from build123d import *

# Parameters (mm, degrees)
CUT_EXTRUDE_START           = 11
CUT_EXTRUDE_1_OUTLINE_R     = 2.9
CUT_EXTRUDE_1_DEPTH         = 5
CUT_EXTRUDE_1_2_OUTLINE_R   = 2.9
CUT_EXTRUDE_1_2_DEPTH       = 4.9999999
CUT_EXTRUDE_START_2         = 2
CUT_EXTRUDE_1_3_OUTLINE_R   = 2.9
CUT_EXTRUDE_1_3_OUTLINE_R_2 = 1.6
CUT_EXTRUDE_1_3_DEPTH       = 12
CUT_EXTRUDE_START_3         = 4.9999999
CUT_EXTRUDE_1_4_OUTLINE_R   = 2.9
CUT_EXTRUDE_1_4_DEPTH       = 6.0000001
CUT_EXTRUDE_START_4         = 15.5
CUT_EXTRUDE_1_5_OUTLINE_R   = 5.75
CUT_EXTRUDE_1_5_OUTLINE_R_2 = 3
CUT_EXTRUDE_1_5_DEPTH       = 1.5
CUT_EXTRUDE_START_5         = 14
CUT_EXTRUDE_1_6_OUTLINE_R   = 4
CUT_EXTRUDE_1_6_OUTLINE_R_2 = 3
CUT_EXTRUDE_1_6_DEPTH       = 1.5
CUT_EXTRUDE_1_7_OUTLINE_R   = 3
CUT_EXTRUDE_1_7_DEPTH       = 14
CUT_EXTRUDE_START_6         = 14.5
CUT_EXTRUDE_1_8_OUTLINE_R   = 3
CUT_EXTRUDE_1_8_DEPTH       = 14
SKETCH_2_R                  = 6.172348418
CUT_EXTRUDE_2_DEPTH         = 3
SKETCH_3_R                  = 1.803021439
CUT_EXTRUDE_3_DEPTH         = 10
SM_BASE_FLANGE_1_DEPTH      = 16
SKETCH_7_R                  = 1.782386215
EXTRUDE_1_DEPTH             = 25
SKETCH_8_R                  = 3.028561668
EXTRUDE_2_DEPTH             = 5
CUT_EXTRUDE_4_DEPTH         = 4
EXTRUDE_3_DEPTH             = 3
SKETCH_11_R                 = 2.38049646
EXTRUDE_4_DEPTH             = 10


with BuildPart() as part:
    # Cut-Extrude 1: read off the stored shape, not the designer's step
    # Cut-Extrude 1 outline → Cut-Extrude 1 (new body)
    with BuildSketch(Plane(origin=(0, 0, 0), x_dir=(1, 0, 0), z_dir=(0, 1, 0)).offset(CUT_EXTRUDE_START)):
        with BuildLine():
            ThreePointArc((-12, 28.5), (-13.414213562, 27.914213562), (-14, 26.5))
            Line((-14, 26.5), (-14, -26.5))
            ThreePointArc((-14, -26.5), (-13.414213562, -27.914213562), (-12, -28.5))
            Line((-12, -28.5), (12, -28.5))
            ThreePointArc((12, -28.5), (13.414213562, -27.914213562), (14, -26.5))
            Line((14, -26.5), (14, 26.5))
            ThreePointArc((14, 26.5), (13.414213562, 27.914213562), (12, 28.5))
            Line((12, 28.5), (-12, 28.5))
        make_face()
        with Locations((9, -23.5)):
            Circle(CUT_EXTRUDE_1_OUTLINE_R, mode=Mode.SUBTRACT)
        with Locations((9, 23.5)):
            Circle(CUT_EXTRUDE_1_OUTLINE_R, mode=Mode.SUBTRACT)
    extrude(amount=CUT_EXTRUDE_1_DEPTH)



with BuildPart() as body_2:
    # Cut-Extrude 1 2 outline → Cut-Extrude 1 2 (new body)
    with BuildSketch(Plane(origin=(0, 0, 0), x_dir=(1, 0, 0), z_dir=(0, 1, 0))):
        with BuildLine():
            ThreePointArc((-12, 28.5), (-13.414213562, 27.914213562), (-14, 26.5))
            Line((-14, 26.5), (-14, -26.5))
            ThreePointArc((-14, -26.5), (-13.414213562, -27.914213562), (-12, -28.5))
            Line((-12, -28.5), (12, -28.5))
            ThreePointArc((12, -28.5), (13.414213562, -27.914213562), (14, -26.5))
            Line((14, -26.5), (14, 26.5))
            ThreePointArc((14, 26.5), (13.414213562, 27.914213562), (12, 28.5))
            Line((12, 28.5), (-12, 28.5))
        make_face()
        with Locations((9, -23.5)):
            Circle(CUT_EXTRUDE_1_2_OUTLINE_R, mode=Mode.SUBTRACT)
        with Locations((9, 23.5)):
            Circle(CUT_EXTRUDE_1_2_OUTLINE_R, mode=Mode.SUBTRACT)
    extrude(amount=CUT_EXTRUDE_1_2_DEPTH)


with BuildPart() as part_1:
    add(part.part)

    add(body_2.part)  # Cut-Extrude 1 3 merges body 2
    # Cut-Extrude 1 3 outline → Cut-Extrude 1 3 (add)
    # profile 1 of 2: a face of its own
    with BuildSketch(Plane(origin=(0, 0, 0), x_dir=(1, 0, 0), z_dir=(0, 1, 0)).offset(CUT_EXTRUDE_START_2)):
        with Locations((9, 23.5)):
            Circle(CUT_EXTRUDE_1_3_OUTLINE_R)
        with Locations((9, 23.5)):
            Circle(CUT_EXTRUDE_1_3_OUTLINE_R_2, mode=Mode.SUBTRACT)
    # profile 2 of 2: a face of its own
    with BuildSketch(Plane(origin=(0, 0, 0), x_dir=(1, 0, 0), z_dir=(0, 1, 0)).offset(CUT_EXTRUDE_START_2)):
        with Locations((9, -23.5)):
            Circle(CUT_EXTRUDE_1_3_OUTLINE_R)
        with Locations((9, -23.5)):
            Circle(CUT_EXTRUDE_1_3_OUTLINE_R_2, mode=Mode.SUBTRACT)
    extrude(amount=CUT_EXTRUDE_1_3_DEPTH)

    # Cut-Extrude 1 4 outline → Cut-Extrude 1 4 (add)
    with BuildSketch(Plane(origin=(0, 0, 0), x_dir=(1, 0, 0), z_dir=(0, 1, 0)).offset(CUT_EXTRUDE_START_3)):
        with BuildLine():
            ThreePointArc((-12, 28.5), (-13.414213562, 27.914213562), (-14, 26.5))
            Line((-14, 26.5), (-14, -26.5))
            ThreePointArc((-14, -26.5), (-13.414213562, -27.914213562), (-12, -28.5))
            Line((-12, -28.5), (12, -28.5))
            ThreePointArc((12, -28.5), (13.414213562, -27.914213562), (14, -26.5))
            Line((14, -26.5), (14, 26.5))
            ThreePointArc((14, 26.5), (13.414213562, 27.914213562), (12, 28.5))
            Line((12, 28.5), (-12, 28.5))
        make_face()
        with Locations((9, -23.5)):
            Circle(CUT_EXTRUDE_1_4_OUTLINE_R, mode=Mode.SUBTRACT)
        with Locations((9, 23.5)):
            Circle(CUT_EXTRUDE_1_4_OUTLINE_R, mode=Mode.SUBTRACT)
    extrude(amount=CUT_EXTRUDE_1_4_DEPTH)



with BuildPart() as body_2_2:
    # Cut-Extrude 1 5 outline → Cut-Extrude 1 5 (new body)
    with BuildSketch(Plane.YZ.offset(CUT_EXTRUDE_START_4)):
        with Locations((8, 7.5)):
            Circle(CUT_EXTRUDE_1_5_OUTLINE_R)
        with Locations((8, 7.5)):
            Circle(CUT_EXTRUDE_1_5_OUTLINE_R_2, mode=Mode.SUBTRACT)
    extrude(amount=CUT_EXTRUDE_1_5_DEPTH)


with BuildPart() as part_2:
    add(part_1.part)

    add(body_2_2.part)  # Cut-Extrude 1 6 merges body 2 2
    # Cut-Extrude 1 6 outline → Cut-Extrude 1 6 (add)
    with BuildSketch(Plane.YZ.offset(CUT_EXTRUDE_START_5)):
        with Locations((8, 7.5)):
            Circle(CUT_EXTRUDE_1_6_OUTLINE_R)
        with Locations((8, 7.5)):
            Circle(CUT_EXTRUDE_1_6_OUTLINE_R_2, mode=Mode.SUBTRACT)
    extrude(amount=CUT_EXTRUDE_1_6_DEPTH)

    # Cut-Extrude 1 7 outline → Cut-Extrude 1 7 (cut)
    with BuildSketch(Plane.YZ):
        with Locations((8, 7.5)):
            Circle(CUT_EXTRUDE_1_7_OUTLINE_R)
    extrude(amount=CUT_EXTRUDE_1_7_DEPTH, mode=Mode.SUBTRACT)

    # Cut-Extrude 1 8 outline → Cut-Extrude 1 8 (cut)
    with BuildSketch(Plane.XY.offset(CUT_EXTRUDE_START_6)):
        with Locations((-5, 8)):
            Circle(CUT_EXTRUDE_1_8_OUTLINE_R)
    extrude(amount=CUT_EXTRUDE_1_8_DEPTH, mode=Mode.SUBTRACT)

    # Sketch 2 → Cut-Extrude 2 (cut)
    with BuildSketch(Plane(origin=(17, 0, 0), x_dir=(0, 0, -1), z_dir=(1, 0, 0))):
        with Locations((-7.5, 8)):
            Circle(SKETCH_2_R)
    extrude(amount=-CUT_EXTRUDE_2_DEPTH, mode=Mode.SUBTRACT)

    # Sketch 3 → Cut-Extrude 3 (cut)
    with BuildSketch(Plane(origin=(0, 0, -28.5), x_dir=(-1, 0, 0), z_dir=(0, 0, -1))):
        with Locations((-7.733778242, 7.980270974)):
            Circle(SKETCH_3_R)
    extrude(amount=-CUT_EXTRUDE_3_DEPTH, mode=Mode.SUBTRACT)



with BuildPart() as body_2_3:
    # Sm Base Flange 1: sheet metal written as solids
    # Sketch 4 → Sm Base Flange 1 (new body)
    with BuildSketch(Plane(origin=(0, 0, 0), x_dir=(1, 0, 0), z_dir=(0, 1, 0))):
        with BuildLine():
            Line((-10.853055632, 28.5), (-10.853055632, 40.567762067))
            ThreePointArc((-10.853055632, 40.567762067), (-10.285838624, 41.937145059), (-8.916455632, 42.504362067))
            Line((-8.916455632, 42.504362067), (1.33725023, 42.504362067))
            Line((1.33725023, 42.504362067), (1.33725023, 41.304362067))
            Line((1.33725023, 41.304362067), (-8.916455632, 41.304362067))
            ThreePointArc((-8.916455632, 41.304362067), (-9.437310487, 41.088616922), (-9.653055632, 40.567762067))
            Line((-9.653055632, 40.567762067), (-9.653055632, 28.5))
            Line((-9.653055632, 28.5), (-10.853055632, 28.5))
        make_face()
    extrude(amount=SM_BASE_FLANGE_1_DEPTH)


with BuildPart() as part_3:
    add(part_2.part)

    add(body_2_3.part)  # Extrude 1 merges body 2 3
    # Sketch 7 → Extrude 1 (add)
    with BuildSketch(Plane(origin=(0, 0, -28.5), x_dir=(-1, 0, 0), z_dir=(0, 0, -1))):
        with Locations((4.3798438, 7.940812922)):
            Circle(SKETCH_7_R)
    extrude(amount=EXTRUDE_1_DEPTH)

    # Sketch 8 → Extrude 2 (add)
    with BuildSketch(Plane(origin=(0, 0, -53.5), x_dir=(-1, 0, 0), z_dir=(0, 0, -1))):
        with Locations((4.3798438, 7.940812922)):
            Circle(SKETCH_8_R)
    extrude(amount=EXTRUDE_2_DEPTH)

    # Sketch 9 → Cut-Extrude 4 (cut)
    with BuildSketch(Plane(origin=(0, 0, -58.5), x_dir=(-1, 0, 0), z_dir=(0, 0, -1))):
        Polygon((3.093792683, 8.769117031), (3.01948584, 7.241212038), (4.305536958, 6.412907929), (5.665894918, 7.112508812), (5.74020176, 8.640413805), (4.454150642, 9.468717915), align=None)
    extrude(amount=-CUT_EXTRUDE_4_DEPTH, mode=Mode.SUBTRACT)

    # Sketch 10 → Extrude 3 (add)
    with BuildSketch(Plane(origin=(0, 0, -42.504362067), x_dir=(-1, 0, 0), z_dir=(0, 0, -1))):
        Polygon((7.727133917, 7.012317312), (6.857589643, 10.375403392), (3.510299527, 11.303899001), (1.032553683, 8.869308531), (1.902097957, 5.506222451), (5.249388073, 4.577726842), align=None)
    extrude(amount=EXTRUDE_3_DEPTH)

    # Sketch 11 → Extrude 4 (add)
    with BuildSketch(Plane.ZY.offset(14)):
        with Locations((-17.942443325, 11.739355059)):
            Circle(SKETCH_11_R)
        with Locations((-17.942443325, 4.138043136)):
            Circle(SKETCH_11_R)
    extrude(amount=EXTRUDE_4_DEPTH)


solid = part_3.part
Geometry: final body of the model. Coordinates: model frame, mm. A direction names the side the tool comes from. Give positions to 0.01 mm unless a question says otherwise; leave off trailing zeros. Loops run counter-clockwise (first coordinate to the right, second up) from the corner with the lowest first, then second, coordinate; pieces in that order, holes last. Notation, with made-up numbers: (76.25, 84) - (128.25, 84) arc R30 cw to (128.25, 109) - close; hole circle Ø4 at (3, 41.25). An arc over 180 degrees is marked (long way). Answer as CSV lines item,"result". Start each with the question number.
1. Section A-A, the plane z = 23.5. Return loops of the section in (x, y).
2. Reachability of faces 4 (the face through (-4, 8, -54.5)), 5 (the face through (6.699, 0.986, -21.735)), 6 (the face through (-24, 4, -18)), 7 (the face through (-6.4, 8, -53.5)) from +Z, -Z, +X, -X, +Y, -Y: full face, straight path, thin tool, end or side. Return the list, or none.
3. Section C-C, the plane z = 7.5. Return loops of the section in (x, y).
4. Ray query, L1, parallel to Z at x = 9, y = 15.05; L2, parallel to Z at x = -6, y = 9.75; L3, parallel to X at y = 11.5, z = 23.5. Return the intervals inside material, ascending.
5. Draft query along Y for faces 1 (the face through (10.526, 7.916, -23.981)), 2 (the face through (-7.3, 8.67, -43.98)), 3 (the face through (-5, 8, 14.5)). Return one class per face: released by +Y, released by -Y, zero draft, split by the parting line, or undercut.
6. Section D-D, the plane x = -19. Return loops of the section in (y, z).
7. Section B-B, the plane z = -38.5. Return loops of the section in (x, y).
8. Pin query (flat end, axial travel): P1, Ø8, axis at y = 5.5, z = -48, coming from the +X side; P2, Ø3.5, axis at x = 9, z = 23.5, coming from the +Y side; P3, Ø6, axis at y = 11, z = -33.5, coming from the +X side. Return the tip coordinate at first contact, or that it passes through.
Answers:
1,outline,"(-14, 0) - (6.1, 0) - (6.1, 2) - (7.4, 2) - (7.4, 14) - (6.1, 14) - (6.1, 16) - (-14, 16) - close; (10.6, 2) - (11.9, 2) - (11.9, 0) - (14, 0) - (14, 16) - (11.9, 16) - (11.9, 14) - (10.6, 14) - close; hole circle Ø6 at (-5, 8)"
2,face 4,"-Z"
2,face 5,"-Y"
2,face 6,"+Z, -Z, -X, +Y, -Y"
2,face 7,"none"
3,outline,"(-14, 0) - (14, 0) - (14, 5) - (0, 5) - (0, 11) - (14, 11) - (14, 16) - (-14, 16) - close"
4,L1,"z = -28.5 to -26.4, -20.6 to 20.6, 26.4 to 28.5"
4,L2,"z = -58.5 to -53.5, -45.5 to -41.3, -28.5 to 14.5"
4,L3,"x = -14 to 7.4, 10.6 to 14"
5,face 1,"zero draft"
5,face 2,"released by +Y"
5,face 3,"undercut"
6,outline,"circle Ø4.76 at (4.14, -17.94); circle Ø4.76 at (11.74, -17.94)"
7,outline,"(-10.85, 0) - (-9.65, 0) - (-9.65, 16) - (-10.85, 16) - close; circle Ø3.56 at (-4.38, 7.94)"
8,P1,"stops at x = -1.1"
8,P2,"stops at y = 14"
8,P3,"stops at x = -2.6"
